Geometry check sheet. Reference: the model listing, model coordinates, mm. Face numbers are marked on the shaded views. A direction names the side the tool comes from. Give positions to 0.01 mm unless a question says otherwise; leave off trailing zeros. Write each loop counter-clockwise with the first axis right and the second up, starting at its lowest first coordinate (ties: lowest second). Pieces come first, ordered by that corner, then holes. Notation, with made-up numbers: (9.25, 72.25) -> (27.25, 72.25) arc R33 cw to (27.25, 105.25) -> close; hole circle Ø11 at (75.5, 42). An arc over 180 degrees is marked (long way). Use a Markdown table: item, result. Add a question column.
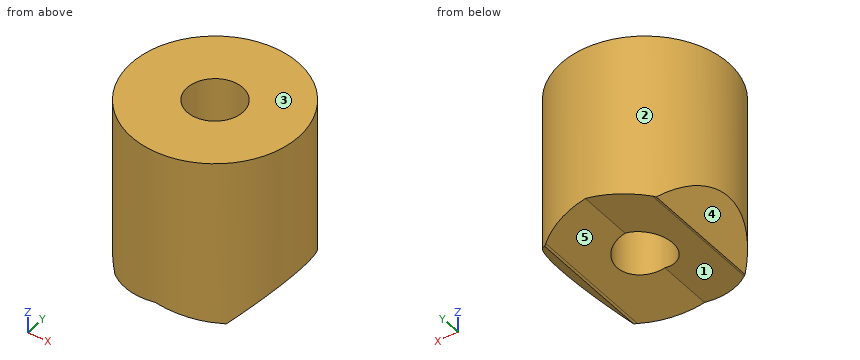
from build123d import *

# Parameters (mm, degrees)
SKETCH1_R               = 38.1
SKETCH1_R_2             = 12.7
BOSS_EXTRUDE1_DEPTH     = 76.2
CUT_EXTRUDE1_DEPTH      = 94.3255592
CUT_EXTRUDE1_DEPTH_BACK = 94.3255592


with BuildPart() as part:
    # Sketch1 → Boss-Extrude1 (new body)
    with BuildSketch(Plane.XY):
        Circle(SKETCH1_R)
        Circle(SKETCH1_R_2, mode=Mode.SUBTRACT)
    extrude(amount=-BOSS_EXTRUDE1_DEPTH)

    # Sketch2 → Cut-Extrude1 (cut, two sides: drawn at the far end of the back side and taken through both)
    with BuildSketch(Plane(origin=(0, 0, 0), x_dir=(1, 0, 0), z_dir=(0, 1, 0)).offset(-CUT_EXTRUDE1_DEPTH_BACK)):
        Polygon((-38.1, 76.2), (-25.4, 76.2), (-38.1, 63.5), align=None)
        with BuildLine():
            Line((0, 76.2), (-25.4, 76.2))
            ThreePointArc((-25.4, 76.2), (-24.878689197, 76.012385142), (-24.339821442, 75.883599159))
            Line((-24.339821442, 75.883599159), (0, 71.4756))
            Line((0, 71.4756), (0, 76.2))
        make_face()
        with BuildLine():
            Line((25.4, 76.2), (0, 76.2))
            Line((0, 76.2), (0, 71.4756))
            Line((0, 71.4756), (24.339821442, 75.883599159))
            ThreePointArc((24.339821442, 75.883599159), (24.878689197, 76.012385142), (25.4, 76.2))
        make_face()
        Polygon((38.1, 76.2), (25.4, 76.2), (38.1, 63.5), align=None)
    extrude(amount=CUT_EXTRUDE1_DEPTH + CUT_EXTRUDE1_DEPTH_BACK, mode=Mode.SUBTRACT)


solid = part.part
1) Draft check along X on the marked faces 3, 4 and 5. Enter one of: +X half, -X half, draft (parallel to the pull), parting line (faces both ways), or undercut.
2) Sectioned sample at B-B, the plane x = 9. Enter the section's corners in (y, z), and give its area (3 significant figures).
3) Sectioned sample at A-A, the plane y = 0. Enter the section's corners in (x, z), and give its area (3 significant figures).
4) Material ranges on probe 1 along X at (y, z) = (0, -45.5); probe 2 along Y at (x, z) = (-4, -35.5), recorded low to high. Write a range as [from, to].
5) Sectioned sample at C-C, the plane y = -15.5. Enter the section's corners in (x, z).
6) Sectioned sample at D-D, the plane z = -8.5. Enter the section's corners in (x, y), and give its area (3 significant figures).
7) Gauge pin test, flat ends, axial feed: P1, Ø1, axis at y = -29, z = -24.5, coming from the -X side; P2, Ø5, axis at y = 27, z = -36, coming from the +X side; P3, Ø2, axis at y = -6, z = -39.5, coming from the -X side. Record the tip position at first contact, or that the pin passes through.
8) Tool access check on the marked faces 1 and 2. Record the directions out of +Z, -Z, +X, -X, +Y, -Y that give a thin tool (end or side, any length) a straight path to the whole face; none if there is none.
Check values:
| question | item | result |
|---|---|---|
| 1 | face 3 | draft |
| 1 | face 4 | -X half |
| 1 | face 5 | undercut |
| 2 | outline | (-37.02, -73.11) -> (-8.96, -73.11) -> (-8.96, 0) -> (-37.02, 0) -> close; (8.96, -73.11) -> (37.02, -73.11) -> (37.02, 0) -> (8.96, 0) -> close |
| 2 | area | 4,100 mm² |
| 3 | outline | (-38.1, -63.5) -> (-25.4, -76.2) arc R5 cw to (-24.34, -75.88) -> (-12.7, -73.78) -> (-12.7, 0) -> (-38.1, 0) -> close; (12.7, -73.78) -> (24.34, -75.88) arc R5 cw to (25.4, -76.2) -> (38.1, -63.5) -> (38.1, 0) -> (12.7, 0) -> close |
| 3 | area | 3,680 mm² |
| 4 | probe 1 | [-38.1, -12.7], [12.7, 38.1] |
| 4 | probe 2 | [-37.89, -12.05], [12.05, 37.89] |
| 5 | outline | (-34.8, -66.8) -> (-25.4, -76.2) arc R5 cw to (-24.34, -75.88) -> (0, -71.48) -> (24.34, -75.88) arc R5 cw to (25.4, -76.2) -> (34.8, -66.8) -> (34.8, 0) -> (-34.8, 0) -> close |
| 6 | outline | circle Ø76.2 at (0, 0); hole circle Ø25.4 at (0, 0) |
| 6 | area | 4,050 mm² |
| 7 | P1 | x = -25.29 |
| 7 | P2 | x = 29.18 |
| 7 | P3 | x = -37.77 |
| 8 | face 1 | -Z, +Y, -Y |
| 8 | face 2 | +Z, -Z |
